Read the model definition and answer for the solid it produces. Units are mm, in the model's axes. A direction names the side the tool comes from. Round coordinates to 2 decimals unless told otherwise and drop trailing zeros. Loops run counter-clockwise (first coordinate to the right, second up) from the corner with the lowest first, then second, coordinate; pieces in that order, holes last. Notation, with made-up numbers: (56, 76) - (72, 76) arc R17 ccw to (72, 105) - close; hole circle Ø4 at (28, 33.25). An arc over 180 degrees is marked (long way). Use one line per item in the form item = value. Start each with the question number.
```python
from build123d import *

# Parameters (mm, degrees)
BOSS_EXTRUDE1_DEPTH = 4.7
SKETCH2_R           = 21
BOSS_EXTRUDE2_DEPTH = 35.3
SKETCH9_R           = 12.5
BOSS_EXTRUDE3_DEPTH = 2
SKETCH10_R          = 5
BOSS_EXTRUDE4_DEPTH = 1
SKETCH11_R          = 4
BOSS_EXTRUDE5_DEPTH = 18
CHAMFER1_SIZE       = 0.5


# Read off the part's stored shape, not the designer's step: Ø3.5 (3.5) Diameter Hole1, Tap Drill for M4x0.7 Tap1
with BuildPart() as part:
    # Sketch1 → Boss-Extrude1 (new body)
    with BuildSketch(Plane.XY):
        Polygon((-21, 17), (-17, 21), (17, 21), (21, 17), (21, -17), (17, -21), (-17, -21), (-21, -17), align=None)
    extrude(amount=BOSS_EXTRUDE1_DEPTH)

    # Sketch2 → Boss-Extrude2 (add)
    with BuildSketch(Plane.XY.offset(4.7)):
        Circle(SKETCH2_R)
    extrude(amount=BOSS_EXTRUDE2_DEPTH)

    # Ø3.5 (3.5) Diameter Hole1 outline → Ø3.5 (3.5) Diameter Hole1 (revolve, cut)
    with BuildSketch(Plane(origin=(-15.5, 15.5, 0), x_dir=(1, 0, 0), z_dir=(0, -1, 0))):
        Polygon((1.75, 0), (1.75, 12), (0.919892113, 12.498779139), (0, 12.498779139), (0, 0), align=None)
    revolve(axis=Axis((-15.5, 15.5, 0), (0, 0, 1)), mode=Mode.SUBTRACT)

    # 3.5 _3.5_ Diameter Hole1 2 outline → 3.5 _3.5_ Diameter Hole1 2 (revolve, cut)
    with BuildSketch(Plane(origin=(15.5, -15.5, 0), x_dir=(1, 0, 0), z_dir=(0, -1, 0))):
        Polygon((1.75, 0), (1.75, 12), (0.919892113, 12.498779139), (0, 12.498779139), (0, 0), align=None)
    revolve(axis=Axis((15.5, -15.5, 0), (0, 0, 1)), mode=Mode.SUBTRACT)

    # 3.5 _3.5_ Diameter Hole1 3 outline → 3.5 _3.5_ Diameter Hole1 3 (revolve, cut)
    with BuildSketch(Plane(origin=(15.5, 15.5, 0), x_dir=(1, 0, 0), z_dir=(0, -1, 0))):
        Polygon((1.75, 0), (1.75, 12), (0.919892113, 12.498779139), (0, 12.498779139), (0, 0), align=None)
    revolve(axis=Axis((15.5, 15.5, 0), (0, 0, 1)), mode=Mode.SUBTRACT)

    # 3.5 _3.5_ Diameter Hole1 4 outline → 3.5 _3.5_ Diameter Hole1 4 (revolve, cut)
    with BuildSketch(Plane(origin=(-15.5, -15.5, 0), x_dir=(1, 0, 0), z_dir=(0, -1, 0))):
        Polygon((1.75, 0), (1.75, 12), (0.919892113, 12.498779139), (0, 12.498779139), (0, 0), align=None)
    revolve(axis=Axis((-15.5, -15.5, 0), (0, 0, 1)), mode=Mode.SUBTRACT)

    # Tap Drill for M4x0.7 Tap1 outline → Tap Drill for M4x0.7 Tap1 (revolve, cut)
    with BuildSketch(Plane(origin=(17.5, 0, 0), x_dir=(1, 0, 0), z_dir=(0, -1, 0))):
        Polygon((0, 40), (0, 31.008579979), (1.65, 32), (1.65, 40), align=None)
    revolve(axis=Axis((17.5, 0, 0), (0, 0, 1)), mode=Mode.SUBTRACT)

    # Tap Drill for M4x0.7 Tap1 2 outline → Tap Drill for M4x0.7 Tap1 2 (revolve, cut)
    with BuildSketch(Plane(origin=(-17.5, 0, 0), x_dir=(1, 0, 0), z_dir=(0, -1, 0))):
        Polygon((0, 40), (0, 31.008579979), (1.65, 32), (1.65, 40), align=None)
    revolve(axis=Axis((-17.5, 0, 0), (0, 0, 1)), mode=Mode.SUBTRACT)

    # Tap Drill for M4x0.7 Tap1 3 outline → Tap Drill for M4x0.7 Tap1 3 (revolve, cut)
    with BuildSketch(Plane.XZ.offset(17.5)):
        Polygon((0, 40), (0, 31.008579979), (1.65, 32), (1.65, 40), align=None)
    revolve(axis=Axis((0, -17.5, 0), (0, 0, 1)), mode=Mode.SUBTRACT)

    # Tap Drill for M4x0.7 Tap1 4 outline → Tap Drill for M4x0.7 Tap1 4 (revolve, cut)
    with BuildSketch(Plane.XZ.offset(-17.5)):
        Polygon((0, 40), (0, 31.008579979), (1.65, 32), (1.65, 40), align=None)
    revolve(axis=Axis((0, 17.5, 0), (0, 0, 1)), mode=Mode.SUBTRACT)

    # Sketch9 → Boss-Extrude3 (add)
    with BuildSketch(Plane.XY.offset(40)):
        Circle(SKETCH9_R)
    extrude(amount=BOSS_EXTRUDE3_DEPTH)

    # Sketch10 → Boss-Extrude4 (add)
    with BuildSketch(Plane.XY.offset(42)):
        Circle(SKETCH10_R)
    extrude(amount=BOSS_EXTRUDE4_DEPTH)

    # Sketch11 → Boss-Extrude5 (add)
    with BuildSketch(Plane.XY.offset(43)):
        Circle(SKETCH11_R)
    extrude(amount=BOSS_EXTRUDE5_DEPTH)

    # Chamfer1
    chamfer1_edges = [part.edges().sort_by_distance(p)[0] for p in [
        (-4, 0, 61),
    ]]
    chamfer(chamfer1_edges, length=CHAMFER1_SIZE)


solid = part.part
```
1) A cutting plane is placed at D-D on z = 49.5. Write down the section's boundary in (x, y).
2) A cutting plane is placed at B-B on z = 6. Write down the section's boundary in (x, y).
3) A cutting plane is placed at C-C on x = -7. Write down the section's boundary in (y, z), plus the area to 3 significant figures.
4) For faces 1 (the cylindrical face through (-14.6, -14, 4.8)), 2 (the flat face through (9, -9, 40)), 3 (the flat face through (0, -21, 2)), 4 (the flat face through (19, -19, 2)), 5 (the flat face through (16, -17.5, 4.7)), determine the directions among +Z, -Z, +X, -X, +Y, -Y from which every point of the face is accessible in a straight line to the end or side of a thin tool.
5) Flat-ended cylindrical pins translate along their axes: pin 1 (23 mm diameter, centred on x = 13.5, y = 9, fed in from +Z); pin 2 (8 mm diameter, centred on x = -8.5, y = 2.5, fed in from -Z); pin 3 (4 mm diameter, centred on x = -6.5, z = 11, fed in from -Y); pin 4 (4 mm diameter, centred on x = 15.5, y = -15.5, fed in from +Z). Find the tip coordinate at first contact, or state that the pin passes through.
6) Straight lines are drawn through the part: line 1 (Y direction, x = 0, z = 35); line 2 (Z direction, x = -14, y = -11); line 3 (Z direction, x = -9, y = 7). For each, find the intervals that lie inside material, in ascending order. Write a range as from..to.
7) A cutting plane is placed at A-A on z = 35.5. Write down the section's boundary in (x, y), plus the area to 3 significant figures.
8) Determine the mould class of faces 6 (the flat face through (-19, -19, 2)), 7 (the flat face through (0, 0, 61)), 8 (the cylindrical face through (14.21, -14.32, 4.75)) for opening direction Y: +Y half, -Y half, draft (parallel to the pull), parting line (faces both ways), or undercut.
Checks:
q1.outline = circle Ø8 at (0, 0)
q2.outline = (-15.84, -13.78) arc R1.75 cw to (-13.78, -15.84) arc R21 ccw to (13.78, -15.84) arc R1.75 cw to (15.84, -13.78) arc R21 ccw to (15.84, 13.78) arc R1.75 cw to (13.78, 15.84) arc R21 ccw to (-13.78, 15.84) arc R1.75 cw to (-15.84, 13.78) arc R21 ccw to start
q3.outline = (-21, 0) - (21, 0) - (21, 4.7) - (19.8, 4.7) - (19.8, 40) - (10.36, 40) - (10.36, 42) - (-10.36, 42) - (-10.36, 40) - (-19.8, 40) - (-19.8, 4.7) - (-21, 4.7) - close
q3.area = 1,640 mm²
q4.face_1 = -Z
q4.face_2 = +Z
q4.face_3 = +Z, -Z, +X, -X, -Y
q4.face_4 = +Z, -Z, +X, -Y
q4.face_5 = +Z, +X, -Y
q5.pin_1 = 43
q5.pin_2 = 0
q5.pin_3 = -20.51
q5.pin_4 = 40
q6.line_1 = -21..-19.15, -15.85..15.85, 19.15..21
q6.line_2 = 0..40
q6.line_3 = 0..42
q7.outline = circle Ø42 at (0, 0); hole circle Ø3.3 at (-17.5, 0); hole circle Ø3.3 at (0, -17.5); hole circle Ø3.3 at (0, 17.5); hole circle Ø3.3 at (17.5, 0)
q7.area = 1,350 mm²
q8.face_6 = -Y half
q8.face_7 = draft
q8.face_8 = undercut
